Source: CAD feature listing. Evaluate the final solid. Frame: model axes, mm. Face numbers are marked on the shaded views. A direction names the side the tool comes from. Coordinates: 2 decimals unless noted, no trailing zeros. Order: outer loops, then holes, each group sorted by start corner. A loop starts at its lowest first (then second) coordinate and runs counter-clockwise, first axis right, second up.
Item 1: Section A-A on y = -7. Return the cut outline in (x, z), then the cut area to 3 significant figures.
Item 2: Section B-B on y = -18. Return the cut outline in (x, z).
Item 3: Section D-D on x = -11.5. State how many separate pieces and enclosed holes the cut face has, then the cut area to 3 significant figures.
Item 4: Ray query, line 1 (Z direction, x = 0, y = 12); line 2 (Y direction, x = -13.9, z = 1.5); line 3 (X direction, y = 3, z = -4.75). Return the intervals inside material, ascending.
Item 5: Contact query for flat-ended pins moving along their axis: P1, Ø5, axis at x = -4.5, z = 6.5, coming from the -Y side; P2, Ø10, axis at x = 12, z = -5.5, coming from the -Y side; P3, Ø7, axis at x = 0, z = -6.5, coming from the +Y side; P4, Ø9, axis at x = 1, z = -8, coming from the -Y side. Output: stop coordinate, or through.
Item 6: Reachability of the marked faces 5, 6 and 7 from +Z, -Z, +X, -X, +Y, -Y: full face, straight path, thin tool, end or side. Return the list, or none.
Item 7: Mould query, pull axis Y, two halves, no side actions, for the marked faces 1, 2, 3 and 4. Classes: released by +Y, released by -Y, zero draft, split by the parting line, or undercut.
Item 8: Section C-C on z = 5.5. Return the cut outline in (x, y), then the cut area to 3 significant figures.
Autodesk Inventor part; units mm, degrees
ref_plane "YZ Plane" through (0, 0, 0) normal (1, 0, 0) x (0, 1, 0)
ref_plane "XZ Plane" through (0, 0, 0) normal (0, 1, 0) x (-1, 0, 0)
ref_plane "XY Plane" through (0, 0, 0) normal (0, 0, 1) x (1, 0, 0)
sketch "Sketch1" plane through (0, 0, 0) normal (0, 0, 1) x (1, 0, 0)
  line L0 (-10, 10.95) -> (10, 10.95)
  line L1 (10, 10.95) -> (10, -10.95)
  line L2 (10, -10.95) -> (-10, -10.95)
  line L3 (-10, -10.95) -> (-10, 10.95)
  line L4 (-15, 15.95) -> (15, 15.95)
  line L5 (15, 15.95) -> (15, -29.05)
  line L6 (15, -29.05) -> (10, -29.05) construction
  line L7 (-15, -29.05) -> (-15, 15.95)
  line L8 (-15, -29.05) -> (-10, -29.05) construction
  line L9 (-10, -29.05) -> (-10, -49.05)
  line L10 (-10, -49.05) -> (-15, -49.05)
  line L11 (-15, -49.05) -> (-15, -29.05)
  line L12 (15, -29.05) -> (10, -29.05) construction
  line L13 (10, -29.05) -> (10, -49.05)
  line L14 (10, -49.05) -> (15, -49.05)
  line L15 (15, -49.05) -> (15, -29.05)
  line L16 (-10, -29.05) -> (-15, -29.05) construction
  line L17 (10, -29.05) -> (-10, -29.05)
  point P0 (0, 0)
  point P1 (0, 10.95)
  point P2 (10, 0)
  dimension "d0" = 20
  dimension "d1" = 21.9
  dimension "d2" = 5
  dimension "d3" = 5
  dimension "d4" = 5
  dimension "d5" = 18.1
  dimension "d6" = 20
extrude "Extrusion1" add sketch "Sketch1" along normal mid plane 27
sketch "Sketch3" plane through (-15, 15.95, 13.5) normal (0, 1, 0) x (1, 0, 0)
  circle A0 centre (15, 20) radius 2.6
  line L0 (0, 27) -> (30, 27)
  point P0 (15, 13.5)
  point P1 (15, 27)
  dimension "d9" = 5.2
  dimension "d10" = 7
extrude "Extrusion2" cut sketch "Sketch3" against normal through all
sketch "Sketch4" plane through (-10, -29.05, 13.5) normal (0, -1, 0) x (1, 0, 0)
  circle A0 centre (10, -20) radius 2.6
  line L0 (14.15, -22.5524) -> (14.15, -17.4476)
  line L1 (14.15, -17.4476) -> (10, -15.35)
  line L2 (10, -15.35) -> (5.85, -17.4476)
  line L3 (5.85, -17.4476) -> (5.85, -22.5524)
  line L4 (5.85, -22.5524) -> (10, -24.65)
  line L5 (10, -24.65) -> (14.15, -22.5524)
  point P0 (10, -13.5)
  point P1 (14.15, -20)
  dimension "d13" = 9.3
  dimension "d14" = 8.3
  dimension "d15" = 8.3
extrude "Extrusion3" cut sketch "Sketch4" against normal blind 14
sketch "Sketch5" plane through (0, 0, 13.5) normal (0, 0, 1) x (1, 0, 0)
  line L0 (10, -29.05) -> (10, -49.05)
  line L1 (-10, -29.05) -> (10, -29.05)
  line L2 (-10, -49.05) -> (-10, -29.05)
  line L3 (10, -29.05) -> (-10, -29.05)
  line L4 (-10, -29.05) -> (-10, -49.05)
  line L5 (-10, -49.05) -> (10, -49.05)
  line L6 (10, -49.05) -> (10, -29.05)
  point P0 (0, 0)
extrude "Extrusion4" add sketch "Sketch5" against normal blind 3
sketch "Sketch6" plane through (15, -49.05, 13.5) normal (1, 0, 0) x (0, 0, -1)
  line L0 (27, 60) -> (27, 38.1)
  line L1 (11, 60) -> (16, 60)
  line L2 (16, 60) -> (16, 48)
  line L3 (16, 48) -> (11, 48)
  line L4 (11, 48) -> (11, 60)
  line L5 (17.4, 65) -> (22.6, 65)
  line L6 (0, 65) -> (27, 65)
  point P0 (13.5, 49.05)
  point P1 (20, 65)
  point P2 (20, 65)
  dimension "d20" = 5
  dimension "d21" = 12
  dimension "d32" = 4
extrude "Extrusion5" cut sketch "Sketch6" against normal up to next
sketch "Sketch7" plane through (-15, -49.05, 13.5) normal (-1, 0, 0) x (0, 0, 1)
  line L0 (-11, 48) -> (-11, 60)
  line L1 (-11, 60) -> (-16, 60)
  line L2 (-16, 60) -> (-16, 48)
  line L3 (-16, 48) -> (-11, 48)
  line L4 (0, 65) -> (-27, 65)
  line L5 (0, 0) -> (0, 65)
  line L6 (0, 0) -> (-27, 0)
  line L7 (-27, 65) -> (-27, 0)
  line L8 (-16, 52.1) -> (-11, 52.1)
  line L9 (-11, 52.1) -> (-11, 40.1)
  line L10 (-11, 40.1) -> (-16, 40.1)
  line L11 (-16, 40.1) -> (-16, 52.1)
  point P0 (-13.5, 49.05)
  point P1 (-27, 38.1)
  dimension "d25" = 5
  dimension "d26" = 12
  dimension "d62" = 2
extrude "Extrusion6" cut sketch "Sketch7" against normal up to next contours L3 L2 L8 L0 | L9 L10 L11 L3
chamfer "Chamfer1" distance 1 angle 45 8 edges at (-12.5, 3.05, 2.5) (-12.5, 3.05, -2.5) (12.5, -1.05, 2.5) (12.5, -1.05, -2.5) (-12.5, -8.95, -2.5) (-12.5, -8.95, 2.5) (12.5, 10.95, 2.5) (12.5, 10.95, -2.5)
sketch "Sketch8" plane through (15, -49.05, 13.5) normal (1, 0, 0) x (0, 0, -1)
  circle A0 centre (12, 10) radius 2.1
  line L0 (0, 0) -> (27, 0)
  point P0 (13.5, 49.05)
  dimension "d33" = 4.2
  dimension "d34" = 10
  dimension "d35" = 15
extrude "Extrusion7" cut sketch "Sketch8" against normal through all
sketch "Sketch9" plane through (0, 0, 13.5) normal (0, 0, 1) x (1, 0, 0)
  line L0 (10, -29.05) -> (-10, -29.05)
  line L1 (10, -49.05) -> (10, -29.05)
  line L2 (10, -49.05) -> (-10, -49.05)
  line L3 (-10, -29.05) -> (-10, -49.05)
  line L4 (-10, -49.05) -> (-7, -40.05)
  line L5 (-7, -40.05) -> (7, -40.05)
  line L6 (10, -49.05) -> (10, -29.05)
  line L7 (7, -40.05) -> (10, -49.05)
  point P0 (0, 0)
  dimension "d38" = 9
  dimension "d39" = 3
extrude "Extrusion8" cut sketch "Sketch9" against normal up to next contours L2 L4 L5 L7
chamfer "Chamfer2" distance 3 angle 45 2 edges at (-7, -40.05, 12) (7, -40.05, 12)
sketch "Sketch10" plane through (-10, -29.05, -13.5) normal (0, -1, 0) x (1, 0, 0)
  line L0 (20, 24) -> (0, 24)
  line L1 (0, 24) -> (0, 0)
  line L2 (20, 0) -> (0, 0)
  line L3 (20, 24) -> (20, 0)
  line L4 (10, 11.65) -> (14.15, 9.5524)
  line L5 (14.15, 9.5524) -> (14.15, 4.4476)
  line L6 (14.15, 4.4476) -> (10, 2.35)
  line L7 (10, 2.35) -> (5.85, 4.4476)
  line L8 (5.85, 4.4476) -> (5.85, 9.5524)
  line L9 (5.85, 9.5524) -> (10, 11.65)
  line L10 (20, 24) -> (0, 24)
  line L11 (0, 24) -> (4, 17.5)
  line L12 (4, 17.5) -> (16, 17.5)
  line L13 (16, 17.5) -> (20, 24)
  point P0 (10, 13.5)
  point P1 (10, 17.5)
  point P2 (10, 24)
  dimension "d45" = 6.5
  dimension "d46" = 12
extrude "Extrusion9" cut sketch "Sketch10" against normal blind 10 contours L13 L12 L11 L0
chamfer "Chamfer3" distance 4 angle 45 2 edges at (6, -24.05, 4) (-6, -24.05, 4)
sketch "Sketch11" plane through (0, 0, -13.5) normal (0, 0, -1) x (-1, 0, 0)
  line L0 (8.0964, -29.05) -> (2, -29.05)
  line L1 (-6.5, -20.05) -> (6.5, -20.05)
  line L2 (6.5, -20.05) -> (6.5, -29.05)
  line L3 (6.5, -29.05) -> (-6.5, -29.05)
  line L4 (-6.5, -29.05) -> (-6.5, -20.05)
  line L5 (-10, -29.05) -> (10, -29.05)
  point P0 (0, 0)
  point P1 (0, -20.05)
  point P2 (0, -29.05)
  dimension "d52" = 13
  dimension "d53" = 9
extrude "Extrusion10" cut sketch "Sketch11" against normal blind 12
sketch "Sketch12" plane through (15, -49.05, 13.5) normal (1, 0, 0) x (0, 0, -1)
  line L0 (0, 0) -> (27, 0)
  line L1 (13, 0) -> (27, 14)
  line L2 (27, 65) -> (27, 0)
  line L3 (22.9, 9.9) -> (27, 21.5)
  point P0 (13.5, 49.05)
  dimension "d56" = 45
  dimension "d57" = 14
  dimension "d58" = 4.1
  dimension "d59" = 7.5
extrude "Extrusion11" cut sketch "Sketch12" against normal through all
sketch "Sketch13" plane through (-15, -49.05, 13.5) normal (-1, 0, 0) x (0, 0, 1)
  line L0 (-16, 41.1) -> (-16, 51.1)
  line L1 (-12, 40.1) -> (-15, 40.1)
  line L2 (-22.9, 9.9) -> (-13, 0)
  line L3 (0, 0) -> (-13, 0)
  line L4 (0, 65) -> (0, 0)
  line L5 (-27, 65) -> (0, 65)
  line L6 (-27, 21.5) -> (-27, 65)
  line L7 (-27, 21.5) -> (-22.9, 9.9)
  circle A0 centre (-12, 10) radius 2.1
  line L8 (-12, 40.1) -> (-15, 40.1)
  line L9 (-16, 41.1) -> (-15, 40.1)
  line L10 (-16, 41.1) -> (-16, 51.1)
  line L11 (-15, 52.1) -> (-16, 51.1)
  line L12 (-15, 52.1) -> (-12, 52.1)
  line L13 (-11, 51.1) -> (-12, 52.1)
  line L14 (-11, 51.1) -> (-11, 41.1)
  line L15 (-12, 40.1) -> (-11, 41.1)
  line L16 (0, 38.1) -> (0, 60)
  line L17 (0, 40.1) -> (-2, 40.1)
  line L18 (-2, 40.1) -> (-2, 52.1)
  line L19 (-2, 52.1) -> (0, 52.1)
  point P0 (-13.5, 49.05)
  dimension "d63" = 2
extrude "Extrusion12" cut sketch "Sketch13" against normal through all contours L17 L18 L19 L4
chamfer "Chamfer4" distance 2 angle 45 4 edges at (-12.5, -8.95, 13.5) (-12.5, 3.05, 13.5) (12.5, -8.95, 13.5) (12.5, 3.05, 13.5)
sketch "Sketch14" plane through (0, 0, 13.5) normal (0, 0, 1) x (1, 0, 0)
  line L0 (-10, 5.05) -> (-10, 10.95)
  line L1 (-10, 5.05) -> (-4.1, 10.95)
  line L2 (10, -0.05) -> (10, 9.95)
  line L3 (-10, 10.95) -> (10, 10.95)
  line L4 (10, 10.95) -> (4.1, 10.95)
  line L5 (10, 5.05) -> (10, 10.95)
  line L6 (4.1, 10.95) -> (10, 5.05)
  point P0 (0, 0)
  dimension "d69" = 45
extrude "Extrusion13" add sketch "Sketch14" against normal blind 4
fillet "Fillet1" radius 2.8 8 edges at (-7.05, 10.95, 9.5) (-10, 8, 9.5) (10, 8, 9.5) (7.05, 10.95, 9.5) (4.1, 10.95, 11.5) (-4.1, 10.95, 11.5) (-10, 5.05, 11.5) (10, 5.05, 11.5)
equation "\"d4\" = d3"
properties part number "holder-GT2-x-carriage-V2-right"
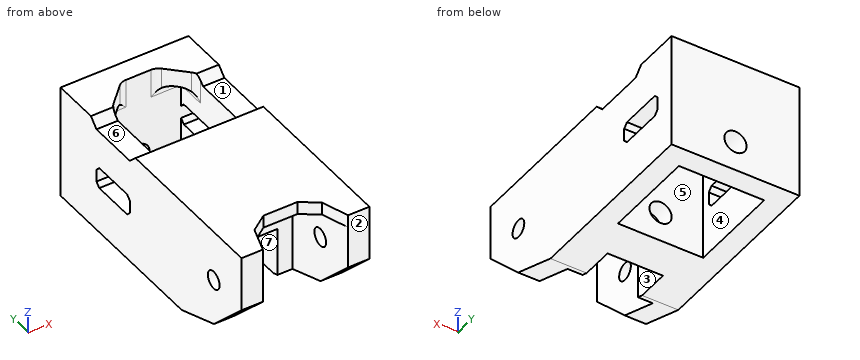
Answer list:
1. outline: (-15, -13.5) - (-10, -13.5) - (-10, -2.5) - (-15, -2.5) - close; (-15, 2.5) - (-10, 2.5) - (-10, 11.5) - (-15, 11.5) - close; (10, -13.5) - (15, -13.5) - (15, 11.5) - (10, 11.5) - close
1. area: 225 mm2
2. outline: (-15, -13.5) - (15, -13.5) - (15, 13.5) - (-15, 13.5) - close; hole (-4.15, -9.05) - (0, -11.15) - (4.15, -9.05) - (4.15, -3.95) - (0, -1.85) - (-4.15, -3.95) - close
3. separate pieces: 1
3. enclosed holes: 2
3. area: 1,540 mm2
4. line 1: z = -13.5 to -9.1, -3.9 to 13.5
4. line 2: y = -49.05 to -41.15, -36.95 to -8.95, 3.05 to 15.95
4. line 3: x = -15 to -10, 10 to 15
5. P1: stops at y = -29.05
5. P2: stops at y = -48.05
5. P3: stops at y = 15.95
5. P4: stops at y = -20.05
6. face 5: +Z, -Z
6. face 6: +Z, +X, -X
6. face 7: -Z, -Y
7. face 1: undercut
7. face 2: released by -Y
7. face 3: zero draft
7. face 4: undercut
8. outline: (-15, -49.05) - (-10, -49.05) - (-10, -29.05) - (-4.68, -29.05) - (-4.68, -19.05) - (4.68, -19.05) - (4.68, -29.05) - (10, -29.05) - (10, -49.05) - (15, -49.05) - (15, 15.95) - (-15, 15.95) - close; hole (-10, -10.95) - (10, -10.95) - (10, 10.95) - (-10, 10.95) - close
8. area: 1,020 mm2
